Job drawing, mm, ordinate dimensions from the low corner. One solid piece. Coordinates: 2 decimals unless noted, no trailing zeros. Write each loop counter-clockwise with the first axis right and the second up, starting at its lowest first coordinate (ties: lowest second). Pieces come first, ordered by that corner, then holes. Notation, with made-up numbers: (27, 82.5) - (42, 82.5) arc R33 ccw to (42, 120.5) - close; hole circle Ø6 at (81.25, 25). An arc over 180 degrees is marked (long way). Use a Markdown table: item, result.
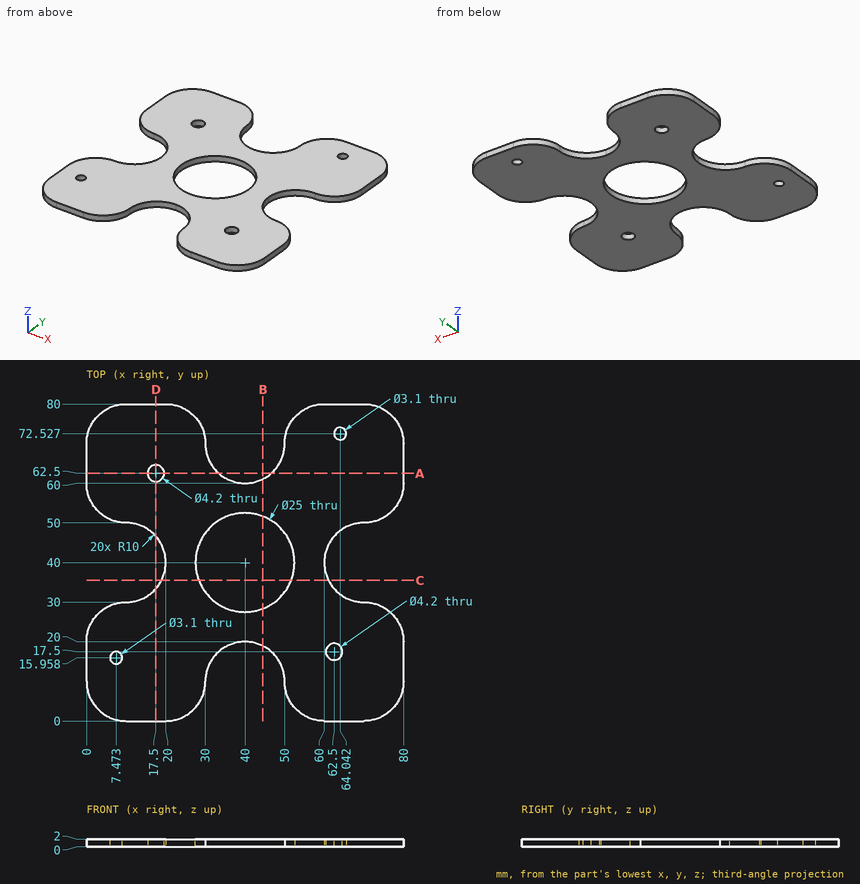
Item 1: Drill centre lines: probe 1 along Y at (x, z) = (17.5, 1.3) (1 decimal); probe 2 along Y at (x, z) = (40, 1.5); probe 3 along X at (y, z) = (40.5, 1.7). Where is each one in solid material? Low to high.
From the geometry:
| item | result |
|---|---|
| probe 1 | 0 to 33.4, 46.6 to 60.4, 64.6 to 80 |
| probe 2 | 20 to 27.5, 52.5 to 60 |
| probe 3 | 19.99 to 27.51, 52.49 to 60.01 |
Item 2: Band-saw the part on B-B, the plane x = 44.5. Give the cut face in (y, z).
From the geometry:
| item | result |
|---|---|
| outline | (18.93, 0) - (28.34, 0) - (28.34, 2) - (18.93, 2) - close; (51.66, 0) - (61.07, 0) - (61.07, 2) - (51.66, 2) - close |
Item 3: Band-saw the part on A-A, the plane y = 62.5. Give the cut face in (x, z) (1 decimal), then the cut area to 3 significant figures.
From the geometry:
| item | result |
|---|---|
| outline | (0, 0) - (15.4, 0) - (15.4, 2) - (0, 2) - close; (19.6, 0) - (33.4, 0) - (33.4, 2) - (19.6, 2) - close; (46.6, 0) - (80, 0) - (80, 2) - (46.6, 2) - close |
| area | 125 mm^2 |
Item 4: Band-saw the part on D-D, the plane x = 17.5. Give the cut face in (y, z) (1 decimal).
From the geometry:
| item | result |
|---|---|
| outline | (0, 0) - (33.4, 0) - (33.4, 2) - (0, 2) - close; (46.6, 0) - (60.4, 0) - (60.4, 2) - (46.6, 2) - close; (64.6, 0) - (80, 0) - (80, 2) - (64.6, 2) - close |
Item 5: Drop flat-ended pins along their axis: P1, Ø2.5, axis at x = 7.47, y = 15.96, coming from the +Z side; P2, Ø1, axis at y = 53.5, z = 1.5, coming from the +X side. Give the stop position or say it passes through.
From the geometry:
| item | result |
|---|---|
| P1 | through |
| P2 | x = 78 |
